Part model, mm, in its own coordinate system. A direction names the side the tool comes from. Round coordinates to 2 decimals unless told otherwise and drop trailing zeros. Loops run counter-clockwise (first coordinate to the right, second up) from the corner with the lowest first, then second, coordinate; pieces in that order, holes last. Notation, with made-up numbers: (46.5, 28) - (92.5, 28) arc R19 ccw to (92.5, 56) - close; hole circle Ø5 at (21, 8.5). An arc over 180 degrees is marked (long way). Write each question's results on one line, items separated by ' | '. Start each with the question number.
(1) Cut at C-C, the plane x = -12.5. List the corners of the cut face in (y, z), then the cut area to 3 significant figures.
(2) Tool access for faces 1 (the face through (-35.966, 0.521, 7.541)), 2 (the face through (-16, -4, 4)), 3 (the face through (-0.66, -1.12, 3.94)): list every direction of +Z, -Z, +X, -X, +Y, -Y with a clear straight run to the whole face (end or side of a thin tool).
(3) Drill centre lines: L1, parallel to X at y = 0, z = 5.75; L2, parallel to Y at x = -32, z = 6.75; L3, parallel to X at y = -1.25, z = 2.5. Where is each one in solid material? Low to high.
(4) Flat gauge pins, fed straight in: P1, Ø4, axis at y = -2.5, z = 7.5, coming from the +X side; P2, Ø2, axis at x = -13, y = 1, coming from the +Z side; P3, Ø1.5, axis at y = 2.5, z = 9.5, coming from the +X side; P4, Ø0.8, axis at y = 0.5, z = 3, coming from the -X side. Where does each tip first touch, or does it go through?
(5) Cut at A-A, the plane y = 0. List the corners of the cut face in (x, z).
(6) Cut at B-B, the plane z = 2. List the corners of the cut face in (x, y).
(7) Cut at D-D, the plane z = 10.5. List the corners of the cut face in (x, y), then the cut area to 3 significant figures.
(8) Mould opens along Y. For faces 4 (the face through (3.966, -0.521, 3.951)), 5 (the face through (0.66, 1.12, 3.94)), 6 (the face through (-14, 0, 8)), 7 (the face through (-0.64, 1.13, 3.94)) say: released by +Y, released by -Y, zero draft, split by the parting line, or undercut.
from build123d import *

# Parameters (mm, degrees)
ESBO_O1_R                = 2
RESSALTO_EXTRUS_O1_DEPTH = 12
ESBO_O2_OUTSIDE_W        = 50.504
ESBO_O2_OUTSIDE_H        = 18.504
ESBO_O2_OUTSIDE_R        = 4
CORTE_EXTRUS_O1_DEPTH    = 1
ESBO_O3_OUTSIDE_W        = 50.504
ESBO_O3_OUTSIDE_H        = 18.504
ESBO_O3_OUTSIDE_R        = 4
CORTE_EXTRUS_O2_DEPTH    = 4
FILETE1_R                = 0.5
CHANFRO1_SIZE            = 0.5


with BuildPart() as part:
    # Esboço1 → Ressalto-extrusão1 (new body)
    with BuildSketch(Plane.XY):
        with BuildLine():
            Line((0, -4), (-32, -4))
            ThreePointArc((-32, -4), (-36, 0), (-32, 4))
            Line((-32, 4), (0, 4))
            ThreePointArc((0, 4), (4, 0), (0, -4))
        make_face()
        with Locations((-32, 0)):
            Circle(ESBO_O1_R, mode=Mode.SUBTRACT)
        Polygon((0, 1.500013734), (-1.29905, 0.750006867), (-1.29905, -0.750006867), (0, -1.500013734), (1.29905, -0.750006867), (1.29905, 0.750006867), align=None, mode=Mode.SUBTRACT)
    extrude(amount=RESSALTO_EXTRUS_O1_DEPTH)

    # Esboço2 outside → Corte-extrusão1 (cut)
    with BuildSketch(Plane(origin=(0, 0, 0), x_dir=(-1, 0, 0), z_dir=(0, 0, -1))):
        with Locations((16, 0)):
            Rectangle(ESBO_O2_OUTSIDE_W, ESBO_O2_OUTSIDE_H)
        with Locations(Location((0, 0, 0), (0, 0, 90))):
            Circle(ESBO_O2_OUTSIDE_R, mode=Mode.SUBTRACT)
    extrude(amount=-CORTE_EXTRUS_O1_DEPTH, mode=Mode.SUBTRACT)

    # Esboço3 outside → Corte-extrusão2 (cut)
    with BuildSketch(Plane.XY.offset(12)):
        with Locations((-16, 0)):
            Rectangle(ESBO_O3_OUTSIDE_W, ESBO_O3_OUTSIDE_H)
        with Locations(Location((-32, 0, 0), (0, 0, 90))):
            Circle(ESBO_O3_OUTSIDE_R, mode=Mode.SUBTRACT)
    extrude(amount=-CORTE_EXTRUS_O2_DEPTH, mode=Mode.SUBTRACT)

    # Filete1
    # the kernel refuses this fillet: 0.5 mm, written as the material it takes off along each edge
    with BuildSketch(Plane(origin=(-32, 0, 12), x_dir=(0, -1, 0), z_dir=(1, 0, 0))) as filete1_piece_1:
        with BuildLine():
            CenterArc((4 - FILETE1_R, FILETE1_R), FILETE1_R, 270, 90)
            Line((4, FILETE1_R), (4, 0))
            Line((4, 0), (4 - FILETE1_R, 0))
        make_face()
    revolve(axis=Axis((-32, 0, 12), (0, 0, -1)), mode=Mode.SUBTRACT)
    with BuildSketch(Plane(origin=(-32, 0, 1), x_dir=(0, -1, 0), z_dir=(1, 0, 0))) as filete1_piece_2:
        with BuildLine():
            CenterArc((4 - FILETE1_R, -FILETE1_R), FILETE1_R, 0, 90)
            Line((4, -FILETE1_R), (4, 0))
            Line((4, 0), (4 - FILETE1_R, 0))
        make_face()
    revolve(axis=Axis((-32, 0, 1), (0, 0, -1)), revolution_arc=180, mode=Mode.SUBTRACT)
    with BuildSketch(Plane(origin=(1.25, 4, 1), x_dir=(0, -1, 0), z_dir=(-1, 0, 0))) as filete1_piece_3_section:
        with BuildLine():
            CenterArc((FILETE1_R, FILETE1_R), FILETE1_R, 180, 90)
            Line((0, FILETE1_R), (0, 0))
            Line((0, 0), (FILETE1_R, 0))
        make_face()
    filete1_piece_3 = extrude(amount=33.25, mode=Mode.PRIVATE)
    filete1_piece_3 = filete1_piece_3 - Plane(origin=(0, 0, 1.115122713), x_dir=(0, 1, 0), z_dir=(0, 0, -1)) * Cylinder(4, 69, mode=Mode.PRIVATE)
    add(filete1_piece_3, mode=Mode.SUBTRACT)
    with BuildSketch(Plane(origin=(-32, -4, 1), x_dir=(0, 0, 1), z_dir=(1, 0, 0))) as filete1_piece_4_section:
        with BuildLine():
            CenterArc((FILETE1_R, -FILETE1_R), FILETE1_R, 90, 90)
            Line((0, -FILETE1_R), (0, 0))
            Line((0, 0), (FILETE1_R, 0))
        make_face()
    filete1_piece_4 = extrude(amount=33.25, mode=Mode.PRIVATE)
    filete1_piece_4 = filete1_piece_4 - Plane(origin=(0, 0, 1.115122438), x_dir=(0, 1, 0), z_dir=(0, 0, -1)) * Cylinder(4, 69, mode=Mode.PRIVATE)
    add(filete1_piece_4, mode=Mode.SUBTRACT)
    with BuildSketch(Plane(origin=(0, 0, 0), x_dir=(0, 1, 0), z_dir=(1, 0, 0))) as filete1_piece_5:
        with BuildLine():
            CenterArc((4 - FILETE1_R, FILETE1_R), FILETE1_R, 270, 90)
            Line((4 - FILETE1_R, 0), (4, 0))
            Line((4, 0), (4, FILETE1_R))
        make_face()
    revolve(axis=Axis((0, 0, 0), (0, 0, 1)), mode=Mode.SUBTRACT)
    with BuildSketch(Plane(origin=(0, 0, 8), x_dir=(0, 1, 0), z_dir=(-1, 0, 0))) as filete1_piece_6:
        with BuildLine():
            CenterArc((4 - FILETE1_R, FILETE1_R), FILETE1_R, 270, 90)
            Line((4 - FILETE1_R, 0), (4, 0))
            Line((4, 0), (4, FILETE1_R))
        make_face()
    revolve(axis=Axis((0, 0, 8), (0, 0, -1)), revolution_arc=180, mode=Mode.SUBTRACT)
    with BuildSketch(Plane(origin=(-33.25, 4, 8), x_dir=(0, 0, -1), z_dir=(1, 0, 0))) as filete1_piece_7_section:
        with BuildLine():
            CenterArc((FILETE1_R, -FILETE1_R), FILETE1_R, 90, 90)
            Line((0, -FILETE1_R), (0, 0))
            Line((0, 0), (FILETE1_R, 0))
        make_face()
    filete1_piece_7 = extrude(amount=33.25, mode=Mode.PRIVATE)
    filete1_piece_7 = filete1_piece_7 - Plane(origin=(-32, 0, 7.884877562), x_dir=(0, -1, 0), z_dir=(0, 0, -1)) * Cylinder(4, 69, mode=Mode.PRIVATE)
    add(filete1_piece_7, mode=Mode.SUBTRACT)
    with BuildSketch(Plane(origin=(0, -4, 8), x_dir=(0, 0, -1), z_dir=(-1, 0, 0))) as filete1_piece_8_section:
        with BuildLine():
            CenterArc((FILETE1_R, -FILETE1_R), FILETE1_R, 90, 90)
            Line((0, -FILETE1_R), (0, 0))
            Line((0, 0), (FILETE1_R, 0))
        make_face()
    filete1_piece_8 = extrude(amount=33.25, mode=Mode.PRIVATE)
    filete1_piece_8 = filete1_piece_8 - Plane(origin=(-32, 0, 7.884877562), x_dir=(0, -1, 0), z_dir=(0, 0, -1)) * Cylinder(4, 69, mode=Mode.PRIVATE)
    add(filete1_piece_8, mode=Mode.SUBTRACT)

    # Chanfro1
    chanfro1_edges = [part.edges().sort_by_distance(p)[0] for p in [
        (-34, 0, 12),
        (-34, 0, 1),
    ]]
    chamfer(chanfro1_edges, length=CHANFRO1_SIZE)


solid = part.part
A:
1) outline: (-4, 1.5) arc R0.5 ccw to (-3.5, 1) - (3.5, 1) arc R0.5 ccw to (4, 1.5) - (4, 7.5) arc R0.5 ccw to (3.5, 8) - (-3.5, 8) arc R0.5 ccw to (-4, 7.5) - close | area: 55.8 mm2
2) face 1: +Z | face 2: +Z, -Z, +X, -X, -Y | face 3: +Z, -Z
3) L1: -36 to -34, -30 to -1.3, 1.3 to 4 | L2: -4 to -2, 2 to 4 | L3: -35.8 to -33.56, -30.44 to -0.43, 0.43 to 3.8
4) P1: x = 3.97 | P2: z = 8 | P3: x = -28.4 | P4: x = -36
5) outline: (-36, 1.5) arc R0.5 ccw to (-35.5, 1) - (-34.5, 1) - (-34, 1.5) - (-34, 11.5) - (-34.5, 12) - (-35.5, 12) arc R0.5 ccw to (-36, 11.5) - close; (-30, 1.5) - (-29.5, 1) - (-4, 1) - (-4, 0.5) arc R0.5 ccw to (-3.5, 0) - (-1.3, 0) - (-1.3, 8) - (-28, 8) - (-28, 11.5) arc R0.5 ccw to (-28.5, 12) - (-29.5, 12) - (-30, 11.5) - close; (1.3, 0) - (3.5, 0) arc R0.5 ccw to (4, 0.5) - (4, 7.5) arc R0.5 ccw to (3.5, 8) - (1.3, 8) - close
6) outline: (-32, -4) - (0, -4) arc R4 ccw to (0, 4) - (-32, 4) arc R4 ccw to start; hole circle Ø4 at (-32, 0); hole (-1.3, -0.75) - (0, -1.5) - (1.3, -0.75) - (1.3, 0.75) - (0, 1.5) - (-1.3, 0.75) - close
7) outline: circle Ø8 at (-32, 0); hole circle Ø4 at (-32, 0) | area: 37.7 mm2
8) face 4: split by the parting line | face 5: undercut | face 6: zero draft | face 7: undercut
